Can you work these out from the drawing? Everything is in mm from the part's minimum corner. Round coordinates to 2 decimals unless told otherwise and drop trailing zeros. Write each loop counter-clockwise with the first axis right and the second up, starting at its lowest first coordinate (ties: lowest second). Pieces come first, ordered by that corner, then holes. Notation, with made-up numbers: (79, 33) -> (130, 33) arc R20 cw to (130, 64) -> close; hole circle Ø9 at (9.25, 28.5). An arc over 180 degrees is marked (long way). Answer as CSV lines item,"result". Start each with the question number.
Q1. Imagine slicing it at A-A on x = 30. Please give me the cut outline in (y, z), and give its area (3 significant figures).
Q2. Imagine slicing it at C-C on y = 74. Please give me the cut outline in (x, z), and give its area (3 significant figures).
Q3. If I drill on line 1 (Y direction, x = 54, z = 26); line 2 (X direction, y = 93.5, z = 27.5); line 3 (Y direction, x = 56.5, z = 38.5), over which ranges is the centre line in solid material (lowest first)? Write a range as [from, to].
Q4. Imagine slicing it at B-B on z = 30. Please give me the cut outline in (x, y).
Q5. Will these pins go through, and if not, where does the flat tip stop? pin 1 Ø3 at (x, y) = (34.5, 123) entering from -Z; pin 2 Ø25 at (x, z) = (40, 26.5) entering from -Y; pin 3 Ø12 at (x, z) = (28, 15.5) entering from -Y; pin 4 Ø8 at (y, z) = (174.5, 19) entering from +X.
Q6. If we mould it in two halves opening along Z, with no side actions, what happens to the marked faces 1 and 2? For each: pulls with the +Z half, pulls with the -Z half, needs draft (parallel to the pull), parting line crosses it, or undercut.
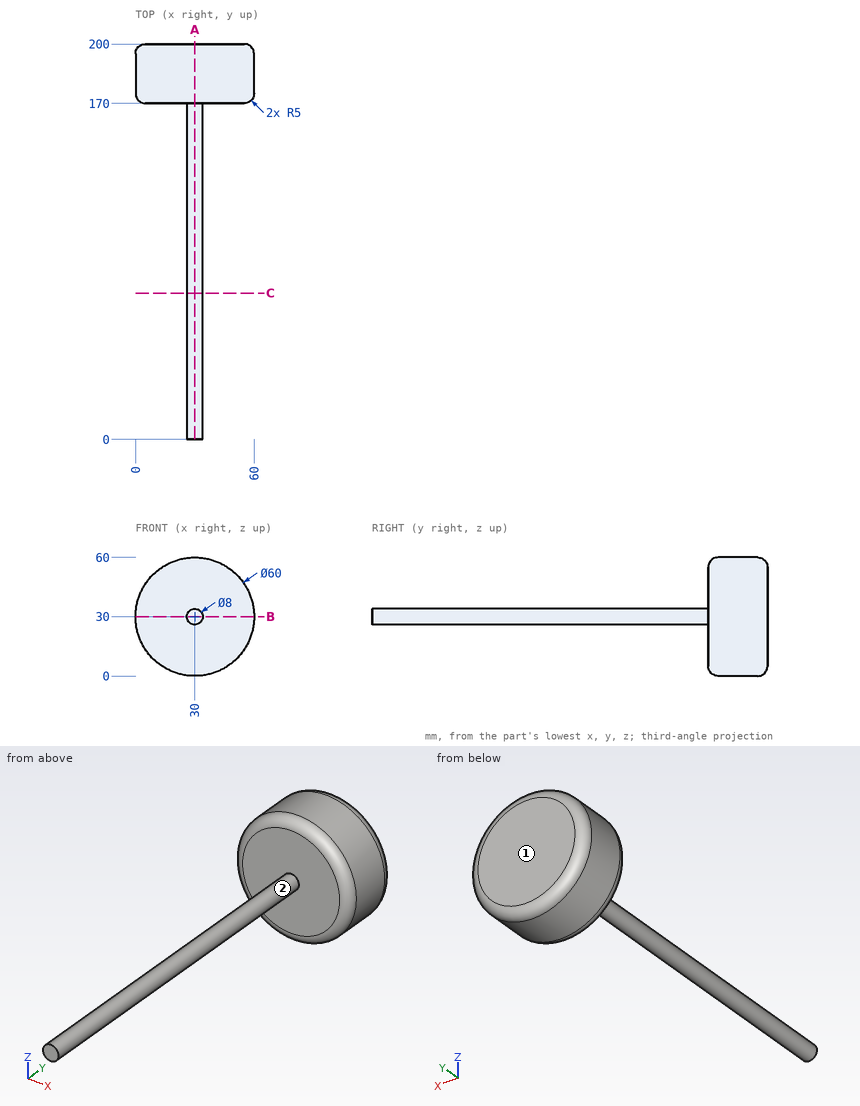
Checks:
1,outline,"(0, 26) -> (170, 26) -> (170, 5) arc R5 ccw to (175, 0) -> (195, 0) arc R5 ccw to (200, 5) -> (200, 55) arc R5 ccw to (195, 60) -> (175, 60) arc R5 ccw to (170, 55) -> (170, 34) -> (0, 34) -> close"
1,area,"3,140 mm^2"
2,outline,"circle Ø8 at (30, 30)"
2,area,"50.3 mm^2"
3,line 1,"[170, 200]"
3,line 2,"[26.88, 33.12]"
3,line 3,"[170.88, 199.12]"
4,outline,"(0, 175) arc R5 ccw to (5, 170) -> (26, 170) -> (26, 0) -> (34, 0) -> (34, 170) -> (55, 170) arc R5 ccw to (60, 175) -> (60, 195) arc R5 ccw to (55, 200) -> (5, 200) arc R5 ccw to (0, 195) -> close"
5,pin 1,"z = 27.35"
5,pin 2,"y = 0"
5,pin 3,"y = 170"
5,pin 4,"x = 59.17"
6,face 1,"needs draft"
6,face 2,"parting line crosses it"
